Design review of the part built by this model. Coordinates are the model's own, in mm. Face numbers are marked on the shaded views. A direction names the side the tool comes from. Round coordinates to 2 decimals unless told otherwise and drop trailing zeros. Order: outer loops, then holes, each group sorted by start corner. A loop starts at its lowest first (then second) coordinate and runs counter-clockwise, first axis right, second up. Notation, with made-up numbers: (88.5, 41.25) - (97.5, 41.25) arc R11 cw to (97.5, 46.25) - close; hole circle Ø10 at (11.25, 15.25). An arc over 180 degrees is marked (long way). Write item = value, one per line.
from build123d import *

# Parameters (mm, degrees)
F1_DEPTH  = 8
F2_R      = 35
F3_DEPTH  = 10
F4_W      = 30
F4_H      = 8
F5_DEPTH  = 8
F6_W      = 60
F6_H      = 2
F7_DEPTH  = 60
F8_W      = 64
F8_H      = 12
F9_DEPTH  = 2
F10_R     = 2.5
F11_DEPTH = 4


# Not quite as in the source:
# - the program builds the solid bodies; features that only make, move or delete a surface that nothing else refers to are left out


with BuildPart() as f1:
    # F0 (on Front) → F1 (new body)
    with BuildSketch(Plane.XZ):
        with BuildLine():
            Line((30, 44.5009035608), (-30, 44.5009035608))
            ThreePointArc((-30, 44.5009035608), (-42.3743686708, 39.3752722315), (-47.5, 27.0009035608))
            Line((-47.5, 27.0009035608), (-47.5, -150.4990964392))
            Line((-47.5, -150.4990964392), (47.5, -150.4990964392))
            Line((47.5, -150.4990964392), (47.5, 27.0009035608))
            ThreePointArc((47.5, 27.0009035608), (42.3743686708, 39.3752722315), (30, 44.5009035608))
        make_face()
    extrude(amount=F1_DEPTH)

    # F2 (on face) → F3 (cut)
    with BuildSketch(Plane.XZ.offset(8)):
        with Locations((0, -35)):
            Circle(F2_R)
    extrude(amount=-F3_DEPTH, mode=Mode.SUBTRACT)

    # F4 (on face) → F5 (cut)
    with BuildSketch(Plane.XZ.offset(8)):
        with Locations((-15, 16.8591848421)):
            Rectangle(F4_W, F4_H)
        with Locations((15, 16.8591848421)):
            Rectangle(F4_W, F4_H)
    extrude(amount=-F5_DEPTH, mode=Mode.SUBTRACT)

    # F6 (on face) → F7 (join)
    with BuildSketch(Plane(origin=(0, 0, 0), x_dir=(-1, 0, 0), z_dir=(0, 1, 0))):
        with Locations((0, 21.8591848421)):
            Rectangle(F6_W, F6_H)
        Polygon((-30, 12.8591848421), (-30, 20.8591848421), (-30, 22.8591848421), (-32, 22.8591848421), (-32, 10.8591848421), (-30, 10.8591848421), align=None)
        Polygon((30, 22.8591848421), (30, 20.8591848421), (30, 12.8591848421), (30, 10.8591848421), (32, 10.8591848421), (32, 22.8591848421), align=None)
        with Locations((0, 11.8591848421)):
            Rectangle(F6_W, F6_H)
    extrude(amount=F7_DEPTH)

    # F8 (on face) → F9 (join)
    with BuildSketch(Plane(origin=(0, 60, 0), x_dir=(-1, 0, 0), z_dir=(0, 1, 0))):
        with Locations((0, 16.8591848421)):
            Rectangle(F8_W, F8_H)
    extrude(amount=F9_DEPTH)

    # F10 (on face) → F11 (cut)
    with BuildSketch(Plane(origin=(0, 0, 10.8591848421), x_dir=(1, 0, 0), z_dir=(0, 0, -1))):
        with Locations((-24.5, -54.5)):
            Circle(F10_R)
    extrude(amount=-F11_DEPTH, mode=Mode.SUBTRACT)


solid = f1.part
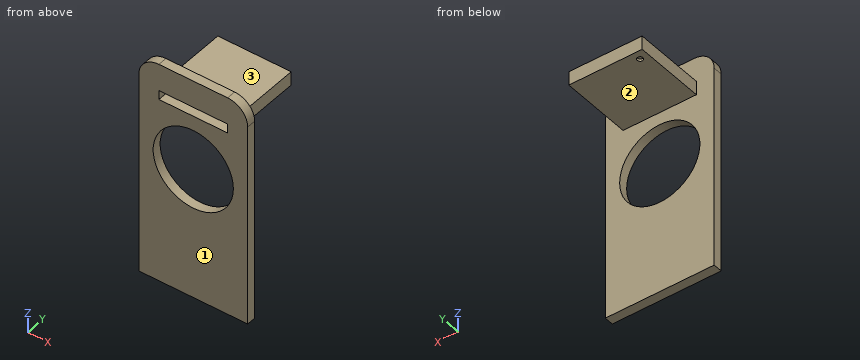
1) We need section A-A on z = -35. Write out the cut boundary in (x, y), and give its area (3 significant figures).
Findings:
outline = (-47.5, -8) - (-35, -8) - (-35, 0) - (-47.5, 0) - close; (35, -8) - (47.5, -8) - (47.5, 0) - (35, 0) - close
area = 200 mm^2
2) We need section C-C on x = -24.5. Write out the cut boundary in (y, z) (3 decimals), and give its area (3 significant figures).
Findings:
outline = (-8, -150.499) - (0, -150.499) - (0, -59.995) - (-8, -59.995) - close; (-8, -10.005) - (0, -10.005) - (0, 10.859) - (52, 10.859) - (52, 12.859) - (-8, 12.859) - close; (-8, 20.859) - (60, 20.859) - (60, 12.859) - (57, 12.859) - (57, 10.859) - (62, 10.859) - (62, 22.859) - (0, 22.859) - (0, 44.501) - (-8, 44.501) - close
area = 1,350 mm^2
3) We need section D-D on y = 54.5. Write out the cut boundary in (x, z), and give its area (3 significant figures).
Findings:
outline = (-32, 10.86) - (-27, 10.86) - (-27, 12.86) - (-30, 12.86) - (-30, 20.86) - (30, 20.86) - (30, 12.86) - (-22, 12.86) - (-22, 10.86) - (32, 10.86) - (32, 22.86) - (-32, 22.86) - close
area = 278 mm^2
4) Clearance check with flat-ended pins moving along their axes: pin 1 Ø6 at (x, y) = (21.5, 26) entering from +Z; pin 2 Ø3.5 at (y, z) = (35, 16) entering from +X; pin 3 Ø18.5 at (x, y) = (7, 28) entering from -Z. State where each tip first meets the part, or that it passes through.
Findings:
pin_1 = 22.86
pin_2 = 32
pin_3 = 10.86
5) For the marked faces 1, 2 and 3, list the 3-axis set-ups (+Z, -Z, +X, -X, +Y, -Y) from which the entire face can be reached by the end or side of a thin tool; tool diameter is ignored.
Findings:
face_1 = +Z, -Z, +X, -X, -Y
face_2 = -Z, +X, -X, +Y
face_3 = +Z, +X, -X, +Y
6) We need section B-B on y = 39.5. Write out the cut boundary in (x, z), and give its area (3 significant figures).
Findings:
outline = (-32, 10.86) - (32, 10.86) - (32, 22.86) - (-32, 22.86) - close; hole (-30, 12.86) - (30, 12.86) - (30, 20.86) - (-30, 20.86) - close
area = 288 mm^2
7) To check wall thickness, follow L1, parallel to Z at x = 0, y = -5; L2, parallel to Z at x = 17, y = 50.5; L3, parallel to X at y = 54.5, z = 12.25. State the ranges of each line that lie inside material, in increasing order. Write a range as from..to.
Findings:
L1 = -150.5..-70, 0..12.86, 20.86..44.5
L2 = 10.86..12.86, 20.86..22.86
L3 = -32..-27, -22..32
